```python
from build123d import *

# Parameters (mm, degrees)
SKETCH_9_R       = 1.6
SKETCH_9_R_2     = 2.5
SKETCH_9_W       = 50
SKETCH_9_H       = 117
EXTRUDE_7_DEPTH  = 3
SKETCH_10_W      = 10
SKETCH_10_H      = 5
EXTRUDE_8_DEPTH  = 30
SKETCH_11_W      = 5
SKETCH_11_H      = 10
EXTRUDE_9_DEPTH  = 20
SKETCH_12_W      = 80
SKETCH_12_H      = 5
EXTRUDE_10_DEPTH = 5
SKETCH_14_W      = 70
SKETCH_14_H      = 5
EXTRUDE_11_DEPTH = 5
CHAMFER_2_SIZE   = 1
CHAMFER_3_SIZE   = 10


with BuildPart() as part:
    # 草图9 → 凸台-拉伸7 (new body)
    with BuildSketch(Plane.XY):
        Polygon((-40, 66.5), (40, 66.5), (40, 10), (72.5, 10), (72.5, -10), (40, -10), (40, -70.5), (-40, -70.5), (-40, -10), (-72.5, -10), (-72.5, 10), (-40, 10), align=None)
        with Locations((25, 61.5)):
            Circle(SKETCH_9_R, mode=Mode.SUBTRACT)
        with Locations((15, -65.5)):
            Circle(SKETCH_9_R, mode=Mode.SUBTRACT)
        with Locations((42.5, 0)):
            Circle(SKETCH_9_R_2, mode=Mode.SUBTRACT)
        with Locations(Location((-42.5, 0, 0), (0, 0, 180))):
            Circle(SKETCH_9_R_2, mode=Mode.SUBTRACT)
        with Locations(Location((-15, -65.5, 0), (0, 0, 180))):
            Circle(SKETCH_9_R, mode=Mode.SUBTRACT)
        with Locations(Location((-25, 61.5, 0), (0, 0, 180))):
            Circle(SKETCH_9_R, mode=Mode.SUBTRACT)
        with Locations((-65, 0)):
            Circle(SKETCH_9_R, mode=Mode.SUBTRACT)
        with Locations((65, 0)):
            Circle(SKETCH_9_R, mode=Mode.SUBTRACT)
        with Locations((0, -2)):
            Rectangle(SKETCH_9_W, SKETCH_9_H, mode=Mode.SUBTRACT)
    extrude(amount=EXTRUDE_7_DEPTH)

    # 草图10 → 凸台-拉伸8 (add)
    with BuildSketch(Plane.XY.offset(3)):
        with Locations((-35, 63)):
            Rectangle(SKETCH_10_W, SKETCH_10_H)
        with Locations((35, 63)):
            Rectangle(SKETCH_10_W, SKETCH_10_H)
    extrude(amount=EXTRUDE_8_DEPTH)

    # 草图11 → 凸台-拉伸9 (add)
    with BuildSketch(Plane.XY.offset(3)):
        with Locations((-32.5, -65.5)):
            Rectangle(SKETCH_11_W, SKETCH_11_H)
        with Locations((32.5, -65.5)):
            Rectangle(SKETCH_11_W, SKETCH_11_H)
    extrude(amount=EXTRUDE_9_DEPTH)

    # 草图12 → 凸台-拉伸10 (add)
    with BuildSketch(Plane.XY.offset(33)):
        with Locations((0, 63)):
            Rectangle(SKETCH_12_W, SKETCH_12_H)
    extrude(amount=-EXTRUDE_10_DEPTH)

    # 草图14 → 凸台-拉伸11 (add)
    with BuildSketch(Plane.XY.offset(23)):
        with Locations((0, -63)):
            Rectangle(SKETCH_14_W, SKETCH_14_H)
    extrude(amount=-EXTRUDE_11_DEPTH)

    # 倒角2
    chamfer_2_edges = [part.edges().sort_by_distance(p)[0] for p in [
        (35, 65.5, 3),
        (-35, 65.5, 3),
        (72.5, -10, 1.5),
        (72.5, 10, 1.5),
        (-72.5, -10, 1.5),
        (-72.5, 10, 1.5),
    ]]
    chamfer(chamfer_2_edges, length=CHAMFER_2_SIZE - 0.0001)  # a hair under: the kernel refuses the full size

    # 倒角3
    chamfer_3_edges = [part.edges().sort_by_distance(p)[0] for p in [
        (40, 10, 1.5),
        (40, -10, 1.5),
        (-40, -10, 1.5),
        (-40, 10, 1.5),
    ]]
    chamfer(chamfer_3_edges, length=CHAMFER_3_SIZE)


solid = part.part
```
Can you work these out from the model? Positions are in its coordinate system, mm. A direction names the side the tool comes from. Coordinates: 2 decimals unless noted, no trailing zeros. Write each loop counter-clockwise with the first axis right and the second up, starting at its lowest first coordinate (ties: lowest second). Pieces come first, ordered by that corner, then holes. Notation, with made-up numbers: M 41,73 L 53,73 A16 ccw 53,88 Z; hole C 85,0 d5. An arc over 180 degrees is marked long. Write item = value, one per line. Start each with the question number.
Q1. On a 3-axis mill with a long thin cutter (end or side, diameter ignored), from which of +Z, -Z, +X, -X, +Y, -Y can I reach the whole of each face in a straight line? I mean faces 1 (the face through (0, 65.5, 29)), 2 (the face through (14.792, -63.914, 1.479)), 3 (the face through (0, -64, 23)). Say none if no direction works.
Q2. If we section it at B-B, the plane y = -18: Write out the boundary of the cut face in (x, z), then the cut area to 3 significant figures.
Q3. If we section it at C-C, the plane x = 42.5: Write out the boundary of the cut face in (y, z).
Q4. I'm going to push flat-ended pins straight in: pin 1 (1.5 mm diameter, centred on y = -33.5, z = 2, fed in from -X); pin 2 (5 mm diameter, centred on y = -65.5, z = 18, fed in from +X); pin 3 (2.5 mm diameter, centred on y = -14, z = 2, fed in from +X); pin 4 (4.5 mm diameter, centred on x = -42.5, y = 0, fed in from -Z). Where does each tip first touch, or does it pass through?
Q5. If I drill on L1, parallel to Y at x = -15, z = 1; L2, parallel to Y at x = -65, z = 2.1; L3, parallel to X at y = -49, z = 2.5, over which ranges is the centre line in solid material (lowest first)? Write a range as [from, to].
Q6. Thinking about a two-plate mould opening in Y: for faces 4 (the face through (-45, 15, 1)), 5 (the face through (-45, -15, 1)), 6 (the face through (-24.792, 59.914, 1.479)), which applies, released by +Y, released by -Y, zero draft, split by the parting line, or undercut?
Q7. If we section it at D-D, the plane z = 7: Write out the boundary of the cut face in (x, y), then the cut area to 3 significant figures.
Q8. If we section it at A-A, the plane x = 1.5: Write out the boundary of the cut face in (y, z).
Check sheet entries:
q1.face_1 = +Z, +X, -X, +Y
q1.face_2 = -Z
q1.face_3 = +Z, +X, -X, -Y
q2.outline = M -42,0 L -25,0 L -25,3 L -42,3 Z; M 25,0 L 42,0 L 42,3 L 25,3 Z
q2.area = 102 mm²
q3.outline = M -17.5,0 L -2.5,0 L -2.5,3 L -17.5,3 Z; M 2.5,0 L 17.5,0 L 17.5,3 L 2.5,3 Z
q4.pin_1 = -40
q4.pin_2 = 35
q4.pin_3 = 47.25
q4.pin_4 = through
q5.L1 = [-70.5, -67.1], [-63.9, -60.5], [56.5, 66.5]
q5.L2 = [-10, -1.6], [1.6, 10]
q5.L3 = [-40, -25], [25, 40]
q6.face_4 = released by +Y
q6.face_5 = released by -Y
q6.face_6 = undercut
q7.outline = M -40,60.5 L -30,60.5 L -30,65.5 L -40,65.5 Z; M -35,-70.5 L -30,-70.5 L -30,-60.5 L -35,-60.5 Z; M 30,-70.5 L 35,-70.5 L 35,-60.5 L 30,-60.5 Z; M 30,60.5 L 40,60.5 L 40,65.5 L 30,65.5 Z
q7.area = 200 mm²
q8.outline = M -70.5,0 L -60.5,0 L -60.5,3 L -70.5,3 Z; M -65.5,18 L -60.5,18 L -60.5,23 L -65.5,23 Z; M 56.5,0 L 66.5,0 L 66.5,3 L 56.5,3 Z; M 60.5,28 L 65.5,28 L 65.5,33 L 60.5,33 Z
